```python
from build123d import *

# Parameters (mm, degrees)
F0_R      = 41.275
F1_DEPTH  = 2.54
F2_R      = 2.54
F3_DEPTH  = 2.541
F4_R      = 2.54
F5_DEPTH  = 2.541
F6_R      = 2.54
F7_DEPTH  = 2.541
F8_R      = 2.54
F9_DEPTH  = 2.541
F10_R     = 1.27
F11_R     = 27.305
F12_DEPTH = 2.541
F13_R     = 20.955
F14_DEPTH = 2.54
F15_R     = 14.605
F16_DEPTH = 2.541
F17_R     = 8.255
F18_DEPTH = 2.54
F19_W     = 3.796444
F19_H     = 24.866691
F20_DEPTH = 2.54
F21_W     = 24.866692
F21_H     = 3.796442
F22_DEPTH = 2.54
F23_W     = 3.796442
F23_H     = 25.815801
F24_DEPTH = 2.54
F25_W     = 24.86669
F25_H     = 3.796442
F26_DEPTH = 2.54


with BuildPart() as f1:
    # F0 (on Top) → F1 (new body)
    with BuildSketch(Plane.XY):
        Circle(F0_R)
    extrude(amount=F1_DEPTH)

    # F2 (on face) → F3 (cut, through all)
    with BuildSketch(Plane.XY.offset(2.54)):
        with Locations((0, 34.925)):
            Circle(F2_R)
    extrude(amount=-F3_DEPTH, mode=Mode.SUBTRACT)

    # F4 (on face) → F5 (cut, through all)
    with BuildSketch(Plane.XY.offset(2.54)):
        with Locations((0, -34.925)):
            Circle(F4_R)
    extrude(amount=-F5_DEPTH, mode=Mode.SUBTRACT)

    # F6 (on face) → F7 (cut, through all)
    with BuildSketch(Plane.XY.offset(2.54)):
        with Locations((-34.925, 0)):
            Circle(F6_R)
    extrude(amount=-F7_DEPTH, mode=Mode.SUBTRACT)

    # F8 (on face) → F9 (cut, through all)
    with BuildSketch(Plane.XY.offset(2.54)):
        with Locations((34.925, 0)):
            Circle(F8_R)
    extrude(amount=-F9_DEPTH, mode=Mode.SUBTRACT)

    # F10
    f10_edges = [f1.edges().sort_by_distance(p)[0] for p in [
        (-41.275, 0, 2.54),
    ]]
    fillet(f10_edges, radius=F10_R)

    # F11 (on face) → F12 (cut, through all)
    with BuildSketch(Plane.XY.offset(2.54)):
        Circle(F11_R)
    extrude(amount=-F12_DEPTH, mode=Mode.SUBTRACT)



with BuildPart() as f14:
    # F13 (on face) → F14 (new body)
    with BuildSketch(Plane.XY.offset(2.54)):
        Circle(F13_R)
    extrude(amount=-F14_DEPTH)

    # F15 (on face) → F16 (cut, through all)
    with BuildSketch(Plane.XY.offset(2.54)):
        Circle(F15_R)
    extrude(amount=-F16_DEPTH, mode=Mode.SUBTRACT)


with BuildPart() as f18:
    # F17 (on face) → F18 (new body)
    with BuildSketch(Plane.XY.offset(2.54)):
        Circle(F17_R)
    extrude(amount=-F18_DEPTH)


with BuildPart() as f1_1:
    add(f1.part)

    add(f14.part)  # F20 merges F14

    add(f18.part)  # F20 merges F18
    # F19 (on face) → F20 (join)
    with BuildSketch(Plane.XY.offset(2.54)):
        with Locations((0, -17.463631)):
            Rectangle(F19_W, F19_H)
    extrude(amount=-F20_DEPTH)

    # F21 (on face) → F22 (join)
    with BuildSketch(Plane.XY.offset(2.54)):
        with Locations((16.989075, -0.094911)):
            Rectangle(F21_W, F21_H)
    extrude(amount=-F22_DEPTH)

    # F23 (on face) → F24 (join)
    with BuildSketch(Plane.XY.offset(2.54)):
        with Locations((0, 17.178897)):
            Rectangle(F23_W, F23_H)
    extrude(amount=-F24_DEPTH)

    # F25 (on face) → F26 (join)
    with BuildSketch(Plane.XY.offset(2.54)):
        with Locations((-18.128007, 0.094911)):
            Rectangle(F25_W, F25_H)
    extrude(amount=-F26_DEPTH)


solid = f1_1.part
```
For this review, take the finished solid that the model builds, in its own axes (mm). Coordinates: 2 decimals unless noted, no trailing zeros. Order: outer loops, then holes, each group sorted by start corner. A loop starts at its lowest first (then second) coordinate and runs counter-clockwise, first axis right, second up. Notation, with made-up numbers: (85, -6.5) - (100, -6.5) arc R22 ccw to (100, 2.5) - close; hole circle Ø8 at (9, 18.5). An arc over 180 degrees is marked (long way). Answer as a JSON object with one key per item and string values. Group by question number.
1. We need section A-A on x = 0. State the section outline as (y, z) points (3 decimals).
2. We need section C-C on z = 2.1. Give the number of separate pieces and of enclosed holes in the cut face, then the cut area to 3 significant figures.
3. For probe 1 along Y at (x, z) = (0, 0.7) (3 decimals); probe 2 along Y at (x, z) = (4.5, 0.8); probe 3 along Y at (x, z) = (15.5, 0.4), list the stretches that pass through material, from the lowest coordinate up.
4. Clearance check with flat-ended pins moving along their axes: P1, Ø1.3, axis at y = 10.5, z = 2, coming from the -X side; P2, Ø4, axis at x = 0, y = -34.925, coming from the -Z side (3 decimals); P3, Ø0.8, axis at y = -25.5, z = 1.5, coming from the -X side; P4, Ø1.5, axis at y = 14, z = 2, coming from the +X side. State where each tip first meets the part, or that it passes through.
Final values:
{
 "1": {"outline": "(-41.275, 0) - (-37.465, 0) - (-37.465, 2.54) - (-40.005, 2.54) arc R1.27 ccw to (-41.275, 1.27) - close; (-32.385, 0) - (32.385, 0) - (32.385, 2.54) - (-32.385, 2.54) - close; (37.465, 0) - (41.275, 0) - (41.275, 1.27) arc R1.27 ccw to (40.005, 2.54) - (37.465, 2.54) - close"},
 "2": {"separate pieces": "1", "enclosed holes": "12", "area": "3,970 mm²"},
 "3": {"probe 1": "-41.275 to -37.465, -32.385 to 32.385, 37.465 to 41.275", "probe 2": "-41.03 to -26.93, -20.47 to -13.89, -6.92 to 6.92, 13.89 to 20.47, 26.93 to 41.03", "probe 3": "-38.25 to -22.48, -14.1 to 14.1, 22.48 to 38.25"},
 "4": {"P1": "x = -40.01", "P2": "through", "P3": "x = -32.75", "P4": "x = 39.01"}
}
